Verification items for the finished model (mm, model axes). Face numbers are marked on the shaded views. Give positions to 0.01 mm unless a question says otherwise; leave off trailing zeros. Write each loop counter-clockwise with the first axis right and the second up, starting at its lowest first coordinate (ties: lowest second). Pieces come first, ordered by that corner, then holes.
from build123d import *

# Parameters (mm, degrees)
SKIZZE1_W                       = 285
SKIZZE1_H                       = 1098
BASIS_LINEAR_AUSTRAGEN_DEPTH    = 23
WANDUNG1_T                      = -2
VERRUNDUNG1_R                   = 2
SCHNITT_LINEAR_AUSTRAGEN1_REACH = 1109.447
SCHNITT_LINEAR_AUSTRAGEN2_REACH = 1109.447


with BuildPart() as part:
    # Skizze1 → Basis-Linear austragen (new body)
    with BuildSketch(Plane.XY):
        with Locations((0, 549)):
            Rectangle(SKIZZE1_W, SKIZZE1_H)
    extrude(amount=-BASIS_LINEAR_AUSTRAGEN_DEPTH)

    # Wandung1
    wandung1_openings = [part.faces().sort_by_distance(p)[0] for p in [
        (0, 549, -23),
    ]]
    offset(amount=WANDUNG1_T, openings=wandung1_openings, kind=Kind.INTERSECTION)

    # Verrundung1
    verrundung1_edges = [part.edges().sort_by_distance(p)[0] for p in [
        (0, 1098, 0),
        (142.5, 549, 0),
        (0, 0, 0),
        (-142.5, 549, 0),
        (-142.5, 1098, -11.5),
        (142.5, 1098, -11.5),
        (142.5, 0, -11.5),
        (-142.5, 0, -11.5),
    ]]
    fillet(verrundung1_edges, radius=VERRUNDUNG1_R)

    # Skizze2 → Schnitt-Linear austragen1 (cut, up to next)
    with BuildSketch(Plane.XY, mode=Mode.PRIVATE) as schnitt_linear_austragen1_sk1:
        with BuildLine():
            Line((-92.555689864, 1053.05), (-82.444310136, 1053.05))
            ThreePointArc((-82.444310136, 1053.05), (-79.545048712, 1050.954951288), (-77.45, 1048.055689864))
            Line((-77.45, 1048.055689864), (-77.45, 1037.944310136))
            ThreePointArc((-77.45, 1037.944310136), (-79.545048712, 1035.045048712), (-82.444310136, 1032.95))
            Line((-82.444310136, 1032.95), (-92.555689864, 1032.95))
            ThreePointArc((-92.555689864, 1032.95), (-95.454951288, 1035.045048712), (-97.55, 1037.944310136))
            Line((-97.55, 1037.944310136), (-97.55, 1048.055689864))
            ThreePointArc((-97.55, 1048.055689864), (-95.454951288, 1050.954951288), (-92.555689864, 1053.05))
        make_face()
    schnitt_linear_austragen1_tool1 = extrude(schnitt_linear_austragen1_sk1.sketch, amount=-SCHNITT_LINEAR_AUSTRAGEN1_REACH, mode=Mode.PRIVATE) & part.part
    schnitt_linear_austragen1 = schnitt_linear_austragen1_tool1.solids().sort_by_distance((-87.5, 1043, 0))[0]
    add(schnitt_linear_austragen1, mode=Mode.SUBTRACT)

    # Skizze3 → Schnitt-Linear austragen2 (cut, up to next)
    with BuildSketch(Plane.XZ, mode=Mode.PRIVATE) as schnitt_linear_austragen2_sk1:
        with BuildLine():
            Line((-89.5, -7.9), (-79.7, -7.9))
            ThreePointArc((-79.7, -7.9), (-76.6, -11), (-79.7, -14.1))
            Line((-79.7, -14.1), (-89.5, -14.1))
            ThreePointArc((-89.5, -14.1), (-92.6, -11), (-89.5, -7.9))
        make_face()
    schnitt_linear_austragen2_tool1 = extrude(schnitt_linear_austragen2_sk1.sketch, amount=-SCHNITT_LINEAR_AUSTRAGEN2_REACH, mode=Mode.PRIVATE) & part.part
    schnitt_linear_austragen2 = schnitt_linear_austragen2_tool1.solids().sort_by_distance((-84.6, 0, -11))[0]
    add(schnitt_linear_austragen2, mode=Mode.SUBTRACT)

    # Spiegeln1: Schnitt-Linear austragen1, Schnitt-Linear austragen2 across plane
    add(schnitt_linear_austragen1.mirror(Plane(origin=(0, 0, 0), x_dir=(0, 0, 1), z_dir=(1, 0, 0))), mode=Mode.SUBTRACT)
    add(schnitt_linear_austragen2.mirror(Plane(origin=(0, 0, 0), x_dir=(0, 0, 1), z_dir=(1, 0, 0))), mode=Mode.SUBTRACT)


solid = part.part
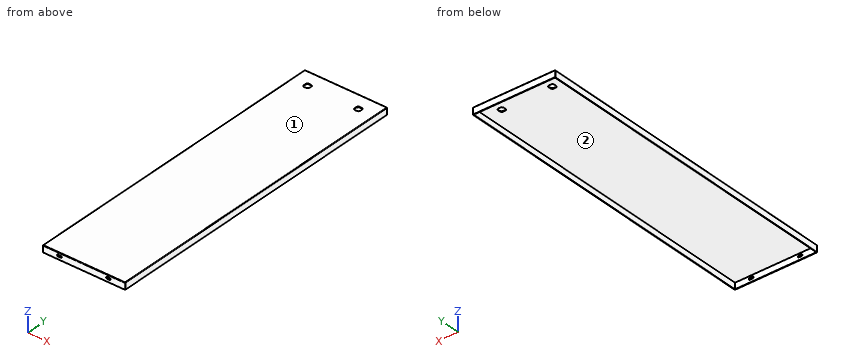
Item 1: Sectioned sample at C-C on x = 8. Record the cut outline in (y, z).
Answer key:
outline: (0, -23) - (2, -23) - (2, -2) - (1096, -2) - (1096, -23) - (1098, -23) - (1098, -2) arc R2 ccw to (1096, 0) - (2, 0) arc R2 ccw to (0, -2) - close
Item 2: Sectioned sample at B-B on y = 333. Record the cut outline in (x, z).
Answer key:
outline: (-142.5, -23) - (-140.5, -23) - (-140.5, -2) - (140.5, -2) - (140.5, -23) - (142.5, -23) - (142.5, -2) arc R2 ccw to (140.5, 0) - (-140.5, 0) arc R2 ccw to (-142.5, -2) - close
Item 3: Depth check by flat-ended pin: pin 1 (0.6 mm diameter, centred on x = 85, y = 1, fed in from +Z); pin 2 (6 mm diameter, centred on x = 113.5, y = 792.5, fed in from -Z); pin 3 (0.6 mm diameter, centred on y = 1040.5, z = -1.5, fed in from +X). Enter the tip coordinate at first touch or a pass-through.
Answer key:
pin 1: stops at z = -0.13
pin 2: stops at z = -2
pin 3: stops at x = 142.49
Item 4: Release check for a two-part mould opening along Y. For the marked faces 1 and 2 record: released by +Y, released by -Y, zero draft, split by the parting line, or undercut.
Answer key:
face 1: zero draft
face 2: undercut
Item 5: Sectioned sample at A-A on z = -19. Record the cut outline in (x, y).
Answer key:
outline: (-142.5, 2) arc R2 ccw to (-140.5, 0) - (140.5, 0) arc R2 ccw to (142.5, 2) - (142.5, 1096) arc R2 ccw to (140.5, 1098) - (-140.5, 1098) arc R2 ccw to (-142.5, 1096) - close; hole (-140.5, 2) - (140.5, 2) - (140.5, 1096) - (-140.5, 1096) - close
Item 6: Scan lines: line 1 along Y through (x, z) = (85, -5.5); line 2 along X through (y, z) = (289, -7.25); line 3 along Z through (x, y) = (65, 536.5). Record each from-to range of solid material in increasing order.
Answer key:
line 1: y = 0 to 2, 1096 to 1098
line 2: x = -142.5 to -140.5, 140.5 to 142.5
line 3: z = -2 to 0
